Build history of the part. All positions in model axes, mm. A direction names the side the tool comes from. Round coordinates to 2 decimals unless told otherwise and drop trailing zeros. Write each loop counter-clockwise with the first axis right and the second up, starting at its lowest first coordinate (ties: lowest second). Pieces come first, ordered by that corner, then holes. Notation, with made-up numbers: (69, 23.25) -> (113, 23.25) arc R21 ccw to (113, 59.25) -> close; hole circle Ø11 at (10, 10.5). An arc over 180 degrees is marked (long way). Return JSON: item names as keys, results as strings.
from build123d import *

# Parameters (mm, degrees)
F0_R     = 17
F0_R_2   = 2.5
F0_R_3   = 7
F1_DEPTH = 5
F0_R_4   = 4
F2_DEPTH = 40
F4_DEPTH = 10


with BuildPart() as f1:
    # F0 (on Front) → F1 (new body)
    with BuildSketch(Plane.XZ):
        Circle(F0_R)
        with Locations((-12, 0)):
            Circle(F0_R_2, mode=Mode.SUBTRACT)
        Circle(F0_R_3, mode=Mode.SUBTRACT)
        with Locations((12, 0)):
            Circle(F0_R_2, mode=Mode.SUBTRACT)
    extrude(amount=F1_DEPTH)

    # F0 (on Front) → F2 (join)
    with BuildSketch(Plane.XZ):
        Circle(F0_R_3)
        Circle(F0_R_4, mode=Mode.SUBTRACT)
    extrude(amount=F2_DEPTH)

    # F3 (on Top) → F4 (cut)
    with BuildSketch(Plane.XY):
        with BuildLine():
            ThreePointArc((0, -32.5), (-1.767767, -36.767767), (2.5, -35))
            ThreePointArc((2.5, -35), (1.767767, -33.232233), (0, -32.5))
        make_face()
    extrude(amount=F4_DEPTH, mode=Mode.SUBTRACT)


solid = f1.part
Q1. Wall check: L1, parallel to Y at x = -9, z = -13; L2, parallel to Y at x = 0, z = 6.05; L3, parallel to Z at x = -12, y = -3.65. Give the ranges that are in metal, low to high.
Verdict:
{"L1": "y = -5 to 0", "L2": "y = -40 to -37.5, -32.5 to 0", "L3": "z = -12.04 to -2.5, 2.5 to 12.04"}
Q2. Two-plate mould, pull along X, no slides. Class faces 3 (the flat face through (7.3, -5, 0.2)), 4 (the cylindrical face through (9.139, -2.465, 14.334)), 5 (the cylindrical face through (-14.5, -2.5, 0.1)): +X half, -X half, draft (parallel to the pull), parting line (faces both ways), or undercut.
Verdict:
{"face 3": "draft", "face 4": "parting line", "face 5": "undercut"}
Q3. Saw through at D-D on x = 1.5. List the corners of the cut face in (y, z).
Verdict:
{"outline": "(-40, -6.84) -> (-5, -6.84) -> (-5, -16.93) -> (0, -16.93) -> (0, -3.71) -> (-40, -3.71) -> close; (-40, 3.71) -> (-37, 3.71) -> (-37, 6.84) -> (-40, 6.84) -> close; (-33, 3.71) -> (0, 3.71) -> (0, 16.93) -> (-5, 16.93) -> (-5, 6.84) -> (-33, 6.84) -> close"}
Q4. 3-axis set-ups, long thin cutter, end or side, ignore diameter. For faces 1 (the cylindrical face through (-1.517, -22.255, -6.834)), 2 (the cylindrical face through (-0.867, -19.72, -3.905)): which of +Z, -Z, +X, -X, +Y, -Y reach the whole face in a straight line?
Verdict:
{"face 1": "-Y", "face 2": "+Y, -Y"}
Q5. Saw through at A-A on z = 0. List the corners of the cut face in (x, y).
Verdict:
{"outline": "(-17, -5) -> (-14.5, -5) -> (-14.5, 0) -> (-17, 0) -> close; (-9.5, -5) -> (-7, -5) -> (-7, -40) -> (-4, -40) -> (-4, 0) -> (-9.5, 0) -> close; (4, -40) -> (7, -40) -> (7, -5) -> (9.5, -5) -> (9.5, 0) -> (4, 0) -> close; (14.5, -5) -> (17, -5) -> (17, 0) -> (14.5, 0) -> close"}
Q6. Saw through at C-C on y = -3.5. List the corners of the cut face in (x, z), then the cut area to 3 significant figures.
Verdict:
{"outline": "circle Ø34 at (0, 0); hole circle Ø5 at (-12, 0); hole circle Ø8 at (0, 0); hole circle Ø5 at (12, 0)", "area": "818 mm²"}
Q7. Pin check, flat tips, straight feed: pin 1 Ø8 at (x, z) = (-2, 6) entering from +Y; pin 2 Ø10 at (y, z) = (-9.5, 8.5) entering from -X; pin 3 Ø2 at (x, y) = (-6, -19) entering from +Z; pin 4 Ø10 at (y, z) = (-30, 3.5) entering from -X. Stop position of each tip, or through.
Verdict:
{"pin 1": "stops at y = 0", "pin 2": "stops at x = -15.78", "pin 3": "stops at z = 4.9", "pin 4": "stops at x = -7"}
Q8. Saw through at B-B on x = 12. List the corners of the cut face in (y, z), then the cut area to 3 significant figures.
Verdict:
{"outline": "(-5, -12.04) -> (0, -12.04) -> (0, -2.5) -> (-5, -2.5) -> close; (-5, 2.5) -> (0, 2.5) -> (0, 12.04) -> (-5, 12.04) -> close", "area": "95.4 mm²"}
